```python
from build123d import *

# Parameters (mm, degrees)
SKETCH_1_W          = 147
SKETCH_1_H          = 50
SKETCH_1_R          = 1.5
EXTRUDE_1_DEPTH     = 2
CUT_EXTRUDE_1_DEPTH = 2
FILLET_2_DEPTH      = 2
FILLET_3_R          = 4
CUT_EXTRUDE_3_DEPTH = 78.661122835
SKETCH_7_R          = 1.75
CUT_EXTRUDE_4_DEPTH = 78.661122835


with BuildPart() as part:
    # 草图1 → 凸台-拉伸1 (new body)
    with BuildSketch(Plane(origin=(0, 0, 0), x_dir=(1, 0, 0), z_dir=(0, 1, 0))):
        Rectangle(SKETCH_1_W, SKETCH_1_H)
        with Locations(Location((18, -18, 0), (0, 0, 270))):
            Circle(SKETCH_1_R, mode=Mode.SUBTRACT)
        with Locations(Location((-18, -18, 0), (0, 0, 270))):
            Circle(SKETCH_1_R, mode=Mode.SUBTRACT)
        with Locations(Location((-18, 18, 0), (0, 0, 270))):
            Circle(SKETCH_1_R, mode=Mode.SUBTRACT)
        with Locations(Location((18, 18, 0), (0, 0, 270))):
            Circle(SKETCH_1_R, mode=Mode.SUBTRACT)
    extrude(amount=EXTRUDE_1_DEPTH)

    # 草图3 → 切除-拉伸1 (cut)
    with BuildSketch(Plane(origin=(0, 2, 0), x_dir=(1, 0, 0), z_dir=(0, 1, 0))):
        with BuildLine():
            Line((-13.345416088, 16.173843213), (0, 2.828427125))
            Line((0, 2.828427125), (13.345416088, 16.173843213))
            ThreePointArc((13.345416088, 16.173843213), (13.868972045, 20.816843629), (18, 23))
            Line((18, 23), (-18, 23))
            ThreePointArc((-18, 23), (-14.464466094, 21.535533906), (-13, 18))
            ThreePointArc((-13, 18), (-13.087112888, 17.070731352), (-13.345416088, 16.173843213))
        make_face()
        with BuildLine():
            Line((16.173843213, 13.345416088), (2.828427125, 0))
            Line((2.828427125, 0), (16.173843213, -13.345416088))
            ThreePointArc((16.173843213, -13.345416088), (20.816843629, -13.868972045), (23, -18))
            Line((23, -18), (23, 18))
            ThreePointArc((23, 18), (20.816843629, 13.868972045), (16.173843213, 13.345416088))
        make_face()
        with BuildLine():
            Line((0, -2.828427125), (-13.345416088, -16.173843213))
            ThreePointArc((-13.345416088, -16.173843213), (-13.087112888, -17.070731352), (-13, -18))
            ThreePointArc((-13, -18), (-14.464466094, -21.535533906), (-18, -23))
            Line((-18, -23), (18, -23))
            ThreePointArc((18, -23), (13.868972045, -20.816843629), (13.345416088, -16.173843213))
            Line((13.345416088, -16.173843213), (0, -2.828427125))
        make_face()
        with BuildLine():
            ThreePointArc((-23, -18), (-20.816843629, -13.868972045), (-16.173843213, -13.345416088))
            Line((-16.173843213, -13.345416088), (-2.828427125, 0))
            Line((-2.828427125, 0), (-16.173843213, 13.345416088))
            ThreePointArc((-16.173843213, 13.345416088), (-20.816843629, 13.868972045), (-23, 18))
            Line((-23, 18), (-23, -18))
        make_face()
    extrude(amount=-CUT_EXTRUDE_1_DEPTH, mode=Mode.SUBTRACT)

    # 圆角2: read off the stored shape, not the designer's step
    # 圆角2 outline → 圆角2 (add)
    with BuildSketch(Plane(origin=(0, 0, 0), x_dir=(1, 0, 0), z_dir=(0, 1, 0))):
        with BuildLine():
            Line((-23, 18), (-23, 9.05572809))
            ThreePointArc((-23, 9.05572809), (-21.666666667, 12.03715206), (-18.555555556, 13.03096005))
            ThreePointArc((-18.555555556, 13.03096005), (-21.726779962, 14.666666667), (-23, 18))
        make_face()
        with BuildLine():
            ThreePointArc((-18.555555556, -13.03096005), (-21.666666667, -12.03715206), (-23, -9.05572809))
            Line((-23, -9.05572809), (-23, -18))
            ThreePointArc((-23, -18), (-21.726779962, -14.666666667), (-18.555555556, -13.03096005))
        make_face()
        with BuildLine():
            ThreePointArc((13.03096005, -18.555555556), (12.03715206, -21.666666667), (9.05572809, -23))
            Line((9.05572809, -23), (18, -23))
            ThreePointArc((18, -23), (14.666666667, -21.726779962), (13.03096005, -18.555555556))
        make_face()
        with BuildLine():
            ThreePointArc((-9.05572809, -23), (-12.03715206, -21.666666667), (-13.03096005, -18.555555556))
            ThreePointArc((-13.03096005, -18.555555556), (-14.666666667, -21.726779962), (-18, -23))
            Line((-18, -23), (-9.05572809, -23))
        make_face()
        with BuildLine():
            ThreePointArc((18.555555556, 13.03096005), (21.666666667, 12.03715206), (23, 9.05572809))
            Line((23, 9.05572809), (23, 18))
            ThreePointArc((23, 18), (21.726779962, 14.666666667), (18.555555556, 13.03096005))
        make_face()
        with BuildLine():
            ThreePointArc((23, -9.05572809), (21.666666667, -12.03715206), (18.555555556, -13.03096005))
            ThreePointArc((18.555555556, -13.03096005), (21.726779962, -14.666666667), (23, -18))
            Line((23, -18), (23, -9.05572809))
        make_face()
        with BuildLine():
            ThreePointArc((-13.03096005, 18.555555556), (-12.03715206, 21.666666667), (-9.05572809, 23))
            Line((-9.05572809, 23), (-18, 23))
            ThreePointArc((-18, 23), (-14.666666667, 21.726779962), (-13.03096005, 18.555555556))
        make_face()
        with BuildLine():
            ThreePointArc((9.05572809, 23), (12.03715206, 21.666666667), (13.03096005, 18.555555556))
            ThreePointArc((13.03096005, 18.555555556), (14.666666667, 21.726779962), (18, 23))
            Line((18, 23), (9.05572809, 23))
        make_face()
    extrude(amount=FILLET_2_DEPTH)

    # 圆角3
    fillet_3_edges = [part.edges().sort_by_distance(p)[0] for p in [
        (13.345416088, 1, 16.173843213),
        (-13.345416088, 1, 16.173843213),
        (0, 1, 2.828427125),
        (16.173843213, 1, -13.345416088),
        (16.173843213, 1, 13.345416088),
        (2.828427125, 1, 0),
        (-16.173843213, 1, -13.345416088),
        (-2.828427125, 1, 0),
        (-16.173843213, 1, 13.345416088),
        (-13.345416088, 1, -16.173843213),
        (13.345416088, 1, -16.173843213),
        (0, 1, -2.828427125),
    ]]
    fillet(fillet_3_edges, radius=FILLET_3_R)

    # 草图6 → 切除-拉伸3 (cut, through all)
    with BuildSketch(Plane(origin=(0, 2, 0), x_dir=(1, 0, 0), z_dir=(0, 1, 0))):
        Polygon((63.5, -25), (56.57179677, -13), (36.57179677, -13), (29.643593539, -25), align=None)
    cut_extrude_3 = extrude(amount=-CUT_EXTRUDE_3_DEPTH, mode=Mode.SUBTRACT)

    # 镜向1: 切除-拉伸3 across plane
    add(cut_extrude_3.mirror(Plane(origin=(0, 0, 0), x_dir=(0, 0, 1), z_dir=(1, 0, 0))), mode=Mode.SUBTRACT)

    # 草图7 → 切除-拉伸4 (cut, through all)
    with BuildSketch(Plane.XZ):
        with Locations(Location((70.5, 20, 0), (0, 0, 270))):
            Circle(SKETCH_7_R)
        with Locations(Location((70.5, -15, 0), (0, 0, 270))):
            Circle(SKETCH_7_R)
        with Locations(Location((-70.5, -15, 0), (0, 0, 270))):
            Circle(SKETCH_7_R)
        with Locations(Location((-70.5, 20, 0), (0, 0, 270))):
            Circle(SKETCH_7_R)
    extrude(amount=-CUT_EXTRUDE_4_DEPTH, mode=Mode.SUBTRACT)


solid = part.part
```
Could you check a few things on this model? Use its own coordinates, in mm. A direction names the side the tool comes from. Give positions to 0.01 mm unless a question says otherwise; leave off trailing zeros. Loops run counter-clockwise (first coordinate to the right, second up) from the corner with the lowest first, then second, coordinate; pieces in that order, holes last. Notation, with made-up numbers: (16, -33) - (41, -33) arc R25 cw to (41, -15) - close; hole circle Ø6 at (-18, -1). An arc over 180 degrees is marked (long way). Answer in a Markdown table with one row per item. Add a question column.
Q1. We'd pull the mould along X, two halves only. Please class faces 1 (the face through (-12.07, 0.99, -21.63)), 2 (the face through (12.07, 0.99, 21.63)), 3 (the face through (-1, 2, 0)): +X half, -X half, draft (parallel to the pull), parting line (faces both ways), or undercut.
Q2. If we section it at B-B (z = 0): List the corners of the cut face in (x, y) for me.
Q3. Please list where these lines run through material, in increasing order: L1, parallel to Z at x = 70.5, y = 1.35; L2, parallel to X at y = 1.35, z = 0; L3, parallel to X at y = 1.95, z = -5.5. Write a range as from..to.
Q4. If we section it at A-A (x = -70.5): List the corners of the cut face in (y, z) for me, plus the area to 3 significant figures.
Q5. If we section it at D-D (y = 1.6): State how many separate pieces and enclosed holes the cut face has, plus the area to 3 significant figures.
Q6. Which directions (+Z, -Z, +X, -X, +Y, -Y) give clear straight access to the entire face, cutting with the end or side of a thin tool? Please do faces 4 (the face through (-7.4, 1.01, -10.23)), 5 (the face through (33.156, 1.014, 18.916)).
Q7. For pin 1 (1 mm diameter, centred on x = -45.5, y = 1, fed in from +Z); pin 2 (3 mm diameter, centred on x = -70.5, z = 20, fed in from -Y), each with a flat end and sliding along its axis, tell me the tip position at first contact or that it passes through.
Q8. If we section it at C-C (z = -7): List the corners of the cut face in (x, y) for me, plus the area to 3 significant figures.
The answers:
| question | item | result |
|---|---|---|
| 1 | face 1 | undercut |
| 1 | face 2 | undercut |
| 1 | face 3 | draft |
| 2 | outline | (-73.5, 0) - (-23, 0) - (-23, 2) - (-73.5, 2) - close; (-4.49, 0) - (4.49, 0) - (4.49, 2) - (-4.49, 2) - close; (23, 0) - (73.5, 0) - (73.5, 2) - (23, 2) - close |
| 3 | L1 | z = -25..-16.75, -13.25..18.25, 21.75..25 |
| 3 | L2 | x = -73.5..-23, -4.49..4.49, 23..73.5 |
| 3 | L3 | x = -73.5..-23, -8.33..-2.66, 2.66..8.33, 23..73.5 |
| 4 | outline | (0, -25) - (2, -25) - (2, -16.75) - (0, -16.75) - close; (0, -13.25) - (2, -13.25) - (2, 18.25) - (0, 18.25) - close; (0, 21.75) - (2, 21.75) - (2, 25) - (0, 25) - close |
| 4 | area | 86.0 mm^2 |
| 5 | separate pieces | 1 |
| 5 | enclosed holes | 12 |
| 5 | area | 5,260 mm^2 |
| 6 | face 4 | +Y, -Y |
| 6 | face 5 | +Z, +Y, -Y |
| 7 | pin 1 | stops at z = 13 |
| 7 | pin 2 | passes through |
| 8 | outline | (-73.5, 0) - (-23, 0) - (-23, 2) - (-73.5, 2) - close; (-9.83, 0) - (-4.17, 0) - (-4.17, 2) - (-9.83, 2) - close; (4.17, 0) - (9.83, 0) - (9.83, 2) - (4.17, 2) - close; (23, 0) - (73.5, 0) - (73.5, 2) - (23, 2) - close |
| 8 | area | 225 mm^2 |
